```python
from build123d import *

# Parameters (mm, degrees)
SKETCH1_W           = 250
SKETCH1_H           = 250
BOSS_EXTRUDE1_DEPTH = 12
SKETCH2_R           = 3.5
CUT_EXTRUDE1_DEPTH  = 3


with BuildPart() as part:
    # Sketch1 → Boss-Extrude1 (new body)
    with BuildSketch(Plane(origin=(0, 0, 0), x_dir=(1, 0, 0), z_dir=(0, 1, 0))):
        Rectangle(SKETCH1_W, SKETCH1_H)
    extrude(amount=BOSS_EXTRUDE1_DEPTH)

    # Sketch2 → Cut-Extrude1 (cut)
    with BuildSketch(Plane.XZ):
        with Locations((-97.5, 45.5)):
            Circle(SKETCH2_R)
        with Locations((-73.5, 45.5)):
            Circle(SKETCH2_R)
        with Locations((-97.5, 27.5)):
            Circle(SKETCH2_R)
        with Locations((-73.5, 27.5)):
            Circle(SKETCH2_R)
        with Locations((-73.5, -27.5)):
            Circle(SKETCH2_R)
        with Locations((-97.5, -27.5)):
            Circle(SKETCH2_R)
        with Locations((-73.5, -45.5)):
            Circle(SKETCH2_R)
        with Locations((-97.5, -45.5)):
            Circle(SKETCH2_R)
        with Locations((97.5, -45.5)):
            Circle(SKETCH2_R)
        with Locations((73.5, -45.5)):
            Circle(SKETCH2_R)
        with Locations((97.5, -27.5)):
            Circle(SKETCH2_R)
        with Locations((73.5, -27.5)):
            Circle(SKETCH2_R)
        with Locations((73.5, 27.5)):
            Circle(SKETCH2_R)
        with Locations((97.5, 27.5)):
            Circle(SKETCH2_R)
        with Locations((73.5, 45.5)):
            Circle(SKETCH2_R)
        with Locations((97.5, 45.5)):
            Circle(SKETCH2_R)
    extrude(amount=-CUT_EXTRUDE1_DEPTH, mode=Mode.SUBTRACT)


solid = part.part
```
The listing builds one solid part. Answer for the finished solid, in the listing's coordinates (mm). A direction names the side the tool comes from. Give positions to 0.01 mm unless a question says otherwise; leave off trailing zeros. Write each loop counter-clockwise with the first axis right and the second up, starting at its lowest first coordinate (ties: lowest second). Pieces come first, ordered by that corner, then holes. Notation, with made-up numbers: M 10.25,-1 L 41.25,-1 A28 ccw 41.25,38 Z; hole C -26,44.25 d11. An arc over 180 degrees is marked long. Write each question's results on one line, items separated by ' | '.
Q1. Section B-B, the plane z = -27.5 is taken. Write down the section's boundary in (x, y).
Output values:
outline: M -125,0 L -101,0 L -101,3 L -94,3 L -94,0 L -77,0 L -77,3 L -70,3 L -70,0 L 70,0 L 70,3 L 77,3 L 77,0 L 94,0 L 94,3 L 101,3 L 101,0 L 125,0 L 125,12 L -125,12 Z
Q2. A tool of negligible diameter and unlimited length cuts with its end or side. For faces 5 (the flat face through (-125, 6, 2)), 6 (the flat face through (97, 3, 28)), from which of +Z, -Z, +X, -X, +Y, -Y can it reach the whole face along a straight path? Write none if from no direction.
Output values:
face 5: +Z, -Z, -X, +Y, -Y | face 6: -Y
Q3. Consider L1, parallel to Z at x = 97.5, y = 1.2. Determine where the line is inside the solid, lowest interval first. Write a range as from..to.
Output values:
L1: -125..-49, -42..-31, -24..24, 31..42, 49..125
Q4. A flat-ended cylindrical pin translates along its axis: P1, Ø3.5, axis at x = -96.5, z = 44.5, coming from the -Y side. Find the tip coordinate at first contact, or state that the pin passes through.
Output values:
P1: y = 3
Q5. For a pull along Z with two mould halves and no side action, classify faces 1 (the flat face through (-2, 6, 125)), 2 (the flat face through (-2, 6, -125)), 3 (the flat face through (-2, 12, -2)), 4 (the flat face through (73, 3, -45)) as released by +Z, released by -Z, zero draft, split by the parting line, or undercut.
Output values:
face 1: released by +Z | face 2: released by -Z | face 3: zero draft | face 4: undercut
Q6. Section A-A, the plane x = 97.5 is taken. Write down the section's boundary in (y, z), then the cut area to 3 significant figures.
Output values:
outline: M 0,-125 L 12,-125 L 12,125 L 0,125 L 0,49 L 3,49 L 3,42 L 0,42 L 0,31 L 3,31 L 3,24 L 0,24 L 0,-24 L 3,-24 L 3,-31 L 0,-31 L 0,-42 L 3,-42 L 3,-49 L 0,-49 Z | area: 2,920 mm2
